from build123d import *

# Parameters (mm, degrees)
F0_R     = 2
F1_DEPTH = 5
F2_R     = 3
F3_DEPTH = 0.6
F5_DEPTH = 2
F6_R     = 10
F7_R     = 2.5


with BuildPart() as f1:
    # F0 (on Top) → F1 (new body)
    with BuildSketch(Plane.XY):
        with BuildLine():
            Line((-58.5, -38.5), (58.5, -38.5))
            ThreePointArc((58.5, -38.5), (62.0355339059, -37.0355339059), (63.5, -33.5))
            Line((63.5, -33.5), (63.5, 33.5))
            ThreePointArc((63.5, 33.5), (62.0355339059, 37.0355339059), (58.5, 38.5))
            Line((58.5, 38.5), (40.2026118555, 38.5))
            ThreePointArc((40.2026118555, 38.5), (37.8876397432, 37.9318059659), (36.0988089683, 36.3563616478))
            ThreePointArc((36.0988089683, 36.3563616478), (0, 17.5), (-36.0988089683, 36.3563616478))
            ThreePointArc((-36.0988089683, 36.3563616478), (-37.8876397432, 37.9318059659), (-40.2026118555, 38.5))
            Line((-40.2026118555, 38.5), (-58.5, 38.5))
            ThreePointArc((-58.5, 38.5), (-62.0355339059, 37.0355339059), (-63.5, 33.5))
            Line((-63.5, 33.5), (-63.5, -33.5))
            ThreePointArc((-63.5, -33.5), (-62.0355339059, -37.0355339059), (-58.5, -38.5))
        make_face()
        with Locations((-57.5, -32.5)):
            Circle(F0_R, mode=Mode.SUBTRACT)
        with Locations((57.5, -32.5)):
            Circle(F0_R, mode=Mode.SUBTRACT)
        with Locations((-57.5, 32.5)):
            Circle(F0_R, mode=Mode.SUBTRACT)
        with Locations((57.5, 32.5)):
            Circle(F0_R, mode=Mode.SUBTRACT)
    extrude(amount=F1_DEPTH)

    # F2 (on face) → F3 (cut)
    with BuildSketch(Plane(origin=(0, 0, 0), x_dir=(1, 0, 0), z_dir=(0, 0, -1))):
        with Locations((-57.5, 32.5)):
            Circle(F2_R)
        with Locations((57.5, 32.5)):
            Circle(F2_R)
        with Locations((57.5, -32.5)):
            Circle(F2_R)
        with Locations((-57.5, -32.5)):
            Circle(F2_R)
    extrude(amount=-F3_DEPTH, mode=Mode.SUBTRACT)

    # F4 (on face) → F5 (cut)
    with BuildSketch(Plane(origin=(0, 0, 0), x_dir=(1, 0, 0), z_dir=(0, 0, -1))):
        Polygon((-8.542372966, 0), (-57.5000000613, 26.5), (-57.5, -26.5), align=None)
        Polygon((-4.0665, 32.5000000613), (-51.5, 32.5000000613), (-4.0665, 6.8249862876), align=None)
        Polygon((51.5, 32.5000000613), (4.0665, 32.5000000613), (4.0665, 6.8249862876), align=None)
        Polygon((57.5000000613, 26.5), (8.542372966, 0), (57.5000000613, -26.5), align=None)
    extrude(amount=-F5_DEPTH, mode=Mode.SUBTRACT)

    # F6
    f6_edges = [f1.edges().sort_by_distance(p)[0] for p in [
        (8.542373, 0, 1),
        (-8.542373, 0, 1),
        (-4.0665, -6.824986, 1),
        (4.0665, -6.824986, 1),
    ]]
    fillet(f6_edges, radius=F6_R)

    # F7
    f7_edges = [f1.edges().sort_by_distance(p)[0] for p in [
        (-51.5, -32.5, 1),
        (51.5, -32.5, 1),
        (57.5, -26.5, 1),
        (57.5, 26.5, 1),
        (-57.5, 26.5, 1),
        (-57.5, -26.5, 1),
        (4.0665, -32.5, 1),
        (-4.0665, -32.5, 1),
    ]]
    fillet(f7_edges, radius=F7_R)


solid = f1.part
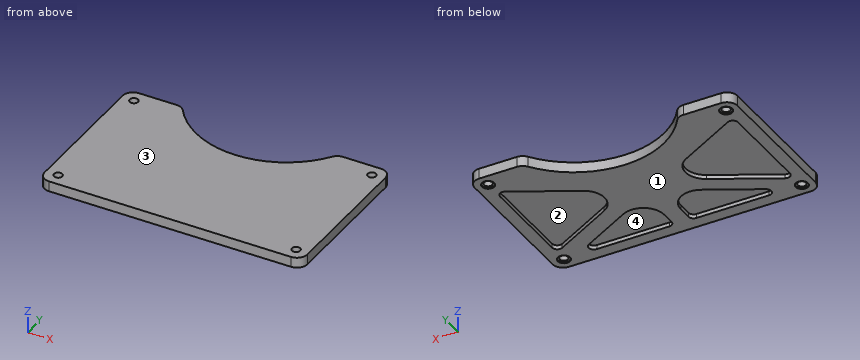
Input: part model. Units: mm. Frame: model coordinates. Face numbers are marked on the shaded views. A direction names the side the tool comes from. Coordinates: 2 decimals unless noted, no trailing zeros. Write each loop counter-clockwise with the first axis right and the second up, starting at its lowest first coordinate (ties: lowest second). Pieces come first, ordered by that corner, then holes. Notation, with made-up numbers: M 87,-16 L 122,-16 A15 cw 122,-11 Z; hole C 74.25,4.25 d4. An arc over 180 degrees is marked long. Answer as a JSON object with one key per item and string values. Group by question number.
(1) Contact query for flat-ended pins moving along their axis: P1, Ø11.5, axis at x = -44.5, y = -12, coming from the -Z side; P2, Ø2, axis at x = -18.5, z = 1, coming from the +Y side; P3, Ø1.8, axis at x = 59, y = -32, coming from the -Z side. Output: stop coordinate, or through.
(2) Section B-B on y = 21. Output: boundary loops of the cut face in (x, z), plus the area to 3 significant figures.
(3) Section C-C on x = 32. Output: boundary loops of the cut face in (y, z), plus the area to 3 significant figures.
(4) Set-up query: the marked faces 3 and 4. Return all of +Z, -Z, +X, -X, +Y, -Y with unobstructed straight access to the full face (end or side cutting, diameter ignored); none if empty.
(5) Section D-D on y = 11. Output: boundary loops of the cut face in (x, z), plus the area to 3 significant figures.
(6) Section A-A on z = 4.15. Output: boundary loops of the cut face in (x, y), plus the area to 3 significant figures.
(7) Ray query, line 1 along X through (y, z) = (-32.5, 3.25); line 2 along Y through (x, z) = (57.5, 2.3); line 3 along X through (y, z) = (32.5, 0.3). Return the intervals inside material, ascending. Write a range as [from, to].
(8) Mould query, pull axis X, two halves, no side actions, for the marked faces 1 and 2. Classes: pulls with the +X half, pulls with the -X half, needs draft (parallel to the pull), parting line crosses it, or undercut.
Result set:
{
 "1": {"P1": "stops at z = 2", "P2": "stops at y = 22.06", "P3": "stops at z = 0.6"},
 "2": {"outline": "M -63.5,0 L -57.5,0 L -57.5,2 L -47.34,2 L -47.34,0 L -17.19,0 L -17.19,5 L -63.5,5 Z; M 17.19,0 L 47.34,0 L 47.34,2 L 57.5,2 L 57.5,0 L 63.5,0 L 63.5,5 L 17.19,5 Z", "area": "422 mm2"},
 "3": {"outline": "M -38.5,0 L -32.5,0 L -32.5,2 L -21.94,2 L -21.94,0 L -12.7,0 L -12.7,2 L 12.7,2 L 12.7,0 L 31.31,0 L 31.31,5 L -38.5,5 Z", "area": "277 mm2"},
 "4": {"face 3": "+Z, +X, -X, +Y, -Y", "face 4": "-Z"},
 "5": {"outline": "M -63.5,0 L -57.5,0 L -57.5,2 L -28.86,2 L -28.86,0 L 28.86,0 L 28.86,2 L 57.5,2 L 57.5,0 L 63.5,0 L 63.5,5 L -63.5,5 Z", "area": "520 mm2"},
 "6": {"outline": "M -63.5,-33.5 A5 ccw -58.5,-38.5 L 58.5,-38.5 A5 ccw 63.5,-33.5 L 63.5,33.5 A5 ccw 58.5,38.5 L 40.2,38.5 A5 ccw 36.1,36.36 A43.98 cw -36.1,36.36 A5 ccw -40.2,38.5 L -58.5,38.5 A5 ccw -63.5,33.5 Z; hole C -57.5,-32.5 d4; hole C -57.5,32.5 d4; hole C 57.5,-32.5 d4; hole C 57.5,32.5 d4", "area": "8,590 mm2"},
 "7": {"line 1": "x = [-63.5, -59.5], [-55.5, 55.5], [59.5, 63.5]", "line 2": "y = [-38.5, -34.5], [-30.5, 30.5], [34.5, 38.5]", "line 3": "x = [-63.5, -60.5], [-54.5, -33.08], [33.08, 54.5], [60.5, 63.5]"},
 "8": {"face 1": "needs draft", "face 2": "undercut"}
}
